```python
from build123d import *

# Parameters (mm, degrees)
BOSS_EXTRUDE1_DEPTH     = 5
SKETCH3_W               = 12
SKETCH3_H               = 5.8
BOSS_EXTRUDE2_DEPTH     = 6
CUT_EXTRUDE1_DEPTH      = 27.191601707
CUT_EXTRUDE1_DEPTH_BACK = 27.191601707
SKETCH4_R               = 1.6
SKETCH5_R               = 2
CUT_EXTRUDE2_DEPTH      = 4
CHAMFER2_SIZE           = 1


with BuildPart() as part:
    # Sketch1 → Boss-Extrude1 (new body)
    with BuildSketch(Plane(origin=(0, 0, 0), x_dir=(1, 0, 0), z_dir=(0, 1, 0))):
        with BuildLine():
            Line((0, 5), (-20, 5))
            ThreePointArc((-20, 5), (-25, 0), (-20, -5))
            Line((-20, -5), (0, -5))
            Line((0, -5), (0, 5))
        make_face()
    extrude(amount=BOSS_EXTRUDE1_DEPTH)

    # Sketch2 → Cut-Revolve1 (revolve, cut)
    with BuildSketch(Plane.XY):
        with BuildLine():
            Line((-20, 1), (-20, 0))
            Line((-20, 0), (-23.31662479, 0))
            ThreePointArc((-23.31662479, 0), (-21.732050808, 0.744562647), (-20, 1))
        make_face()
    revolve(axis=Axis((-20, -4.110143275, 0), (0, 1, 0)), mode=Mode.SUBTRACT)

    # Sketch3 → Boss-Extrude2 (add)
    with BuildSketch(Plane.XZ):
        with Locations((-6, 0)):
            Rectangle(SKETCH3_W, SKETCH3_H)
    extrude(amount=BOSS_EXTRUDE2_DEPTH)

    # Sketch4 → Cut-Extrude1 (cut, two sides: drawn at the far end of the back side and taken through both)
    with BuildSketch(Plane(origin=(0, 0, 0), x_dir=(1, 0, 0), z_dir=(0, 1, 0)).offset(-CUT_EXTRUDE1_DEPTH_BACK)):
        with Locations(Location((-9.210618834, 0, 0), (0, 0, 270))):
            Circle(SKETCH4_R)
    extrude(amount=CUT_EXTRUDE1_DEPTH + CUT_EXTRUDE1_DEPTH_BACK, mode=Mode.SUBTRACT)

    # Sketch5 → Cut-Extrude2 (cut)
    with BuildSketch(Plane(origin=(0, 5, 0), x_dir=(1, 0, 0), z_dir=(0, 1, 0))):
        with Locations(Location((-9.210618834, 0, 0), (0, 0, 270))):
            Circle(SKETCH5_R)
    extrude(amount=-CUT_EXTRUDE2_DEPTH, mode=Mode.SUBTRACT)

    # Mirror1: part across plane


with BuildPart() as part_1:
    add(part.part)
    add(part.part.mirror(Plane(origin=(0, 0, 0), x_dir=(0, 0, 1), z_dir=(1, 0, 0))))

    # Chamfer2
    chamfer2_edges = [part_1.edges().sort_by_distance(p)[0] for p in [
        (0, -6, 2.9),
        (0, -6, -2.9),
        (25, 0, 0),
        (0, 0, 5),
        (-25, 0, 0),
        (0, 0, -5),
    ]]
    chamfer(chamfer2_edges, length=CHAMFER2_SIZE)


solid = part_1.part
```
Geometry check sheet. Reference: the model listing, model coordinates, mm. A direction names the side the tool comes from. Coordinates: 2 decimals unless noted, no trailing zeros. Write each loop counter-clockwise with the first axis right and the second up, starting at its lowest first coordinate (ties: lowest second). Pieces come first, ordered by that corner, then holes. Notation, with made-up numbers: M -22.75,20 L 9.25,20 A14 cw 9.25,33 Z; hole C 25.25,43 d10. An arc over 180 degrees is marked long. Use one line per item in the form item = value. Start each with the question number.
1) Release check for a two-part mould opening along X. For faces 5 (the cylindrical face through (7.228, 3.028, -0.26)), 6 (the flat face through (0, 3, 5)), 7 (the flat face through (12, -3, 0)) record: pulls with the +X half, pulls with the -X half, needs draft (parallel to the pull), parting line crosses it, or undercut.
2) Section check D-D on x = -13.5. Enter the section's corners in (y, z), and give its area (3 significant figures).
3) Section check A-A on z = 0. State how many separate pieces and enclosed holes the cut face has, and give its area (3 significant figures).
4) Go/stop test with flat-tipped pins: pin 1 Ø1.5 at (x, y) = (3, -1.5) entering from -Z; pin 2 Ø3.5 at (x, z) = (-9.21, 0) entering from +Y; pin 3 Ø2.5 at (x, y) = (-4.5, -1.5) entering from +Z; pin 4 Ø3 at (x, z) = (-9.21, 0) entering from -Y. Record where each tip stops, or that it passes through.
5) Thickness scan on probe 1 along X at (y, z) = (-3.5, 0); probe 2 along X at (y, z) = (0.25, 0); probe 3 along X at (y, z) = (2, -0.5). Record the ranges inside material, lowest first. Write a range as from..to.
6) Section check C-C on y = -4.5. Enter the section's corners in (x, z), and give its area (3 significant figures).
7) Section check B-B on x = -0.5. Enter the section's corners in (y, z).
8) Set-up check for faces 1 (the flat face through (0, -2, 2.9)), 2 (the flat face through (-12, -3, 0)), 3 (the flat face through (0, -2, -2.9)), 4 (the cylindrical face through (-7.228, 3.028, -0.26)): record each of +Z, -Z, +X, -X, +Y, -Y from which the full face is reachable in a straight line by a thin tool's end or side.
Responses:
q1.face_5 = undercut
q1.face_6 = needs draft
q1.face_7 = pulls with the +X half
q2.outline = M 0,-4 L 1,-5 L 5,-5 L 5,5 L 1,5 L 0,4 Z
q2.area = 49.0 mm2
q3.separate_pieces = 3
q3.enclosed_holes = 0
q3.area = 307 mm2
q4.pin_1 = -2.9
q4.pin_2 = 1
q4.pin_3 = 2.9
q4.pin_4 = through
q5.probe_1 = -12..-10.81, -7.61..7.61, 10.81..12
q5.probe_2 = -24.25..-22.9, -17.1..-10.81, -7.61..7.61, 10.81..17.1, 22.9..24.25
q5.probe_3 = -24.97..-11.15, -7.27..7.27, 11.15..24.97
q6.outline = M -12,-2.9 L 12,-2.9 L 12,2.9 L -12,2.9 Z; hole C -9.21,0 d3.2; hole C 9.21,0 d3.2
q6.area = 123 mm2
q7.outline = M -6,-1.9 L -5,-2.9 L 0,-2.9 L 0,-4 L 1,-5 L 5,-5 L 5,5 L 1,5 L 0,4 L 0,2.9 L -5,2.9 L -6,1.9 Z
q8.face_1 = +Z, +X, -X, -Y
q8.face_2 = +Z, -Z, -X, -Y
q8.face_3 = -Z, +X, -X, -Y
q8.face_4 = +Y
